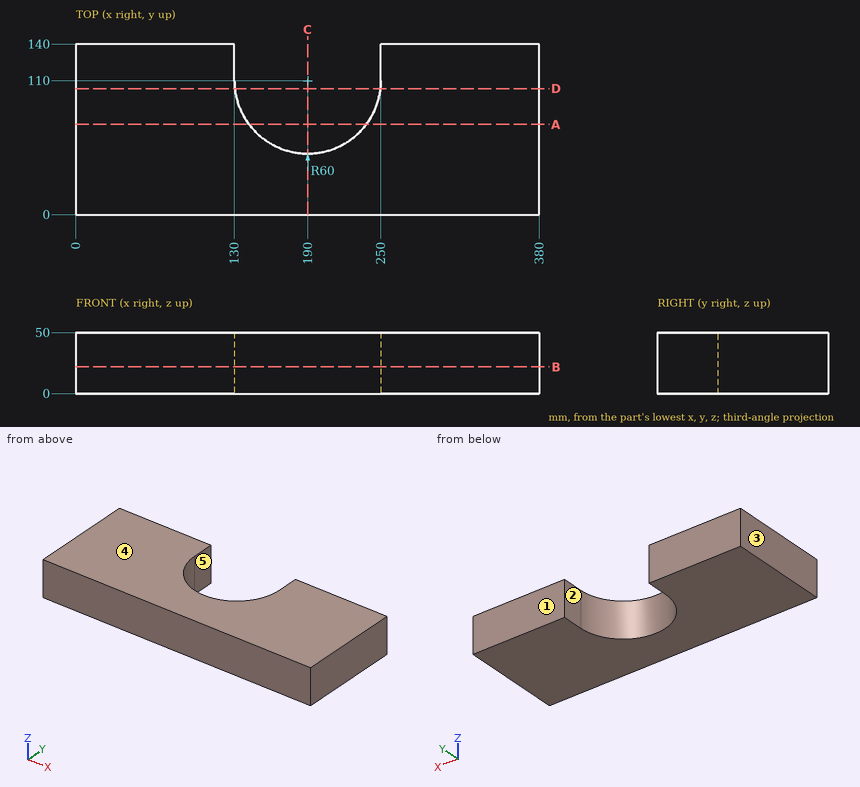
Input: dimensioned drawing with shaded views. Units: mm. Origin: part minimum x, y, z. A direction names the side the tool comes from. Coordinates: 2 decimals unless noted, no trailing zeros. Loops run counter-clockwise (first coordinate to the right, second up) from the corner with the lowest first, then second, coordinate; pieces in that order, holes last. Notation, with made-up numbers: M -32.75,53 L 13.25,53 A16 ccw 13.25,61 Z; hole C 71,48 d10. An arc over 180 degrees is marked long. Use a Markdown table: item, result. Add a question column.
1) Draft query along X for the marked faces 1, 2 and 3. Return one class per face: +X half, -X half, draft (parallel to the pull), parting line (faces both ways), or undercut.
2) Section A-A, the plane y = 74. Return the cut outline in (x, z), plus the area to 3 significant figures.
3) Section B-B, the plane z = 22. Return the cut outline in (x, y), plus the area to 3 significant figures.
4) Section D-D, the plane y = 103.5. Return the cut outline in (x, z), plus the area to 3 significant figures.
5) Set-up query: the marked faces 4 and 5. Return all of +Z, -Z, +X, -X, +Y, -Y with unobstructed straight access to the full face (end or side cutting, diameter ignored); none if empty.
6) Line query: L1, parallel to X at y = 130, z = 42; L2, parallel to X at y = 55, z = 42; L3, parallel to Y at x = 194.5, z = 3. Output: solid intervals per line, ascending. Write a range as from..to.
7) Section C-C, the plane x = 190. Return the cut outline in (y, z), plus the area to 3 significant figures.
Answer below:
| question | item | result |
|---|---|---|
| 1 | face 1 | draft |
| 1 | face 2 | undercut |
| 1 | face 3 | -X half |
| 2 | outline | M 0,0 L 142,0 L 142,50 L 0,50 Z; M 238,0 L 380,0 L 380,50 L 238,50 Z |
| 2 | area | 14,200 mm2 |
| 3 | outline | M 0,0 L 380,0 L 380,140 L 250,140 L 250,110 A60 cw 130,110 L 130,140 L 0,140 Z |
| 3 | area | 43,900 mm2 |
| 4 | outline | M 0,0 L 130.35,0 L 130.35,50 L 0,50 Z; M 249.65,0 L 380,0 L 380,50 L 249.65,50 Z |
| 4 | area | 13,000 mm2 |
| 5 | face 4 | +Z, +X, -X, +Y, -Y |
| 5 | face 5 | +Z, -Z, +Y |
| 6 | L1 | 0..130, 250..380 |
| 6 | L2 | 0..166.02, 213.98..380 |
| 6 | L3 | 0..50.17 |
| 7 | outline | M 0,0 L 50,0 L 50,50 L 0,50 Z |
| 7 | area | 2,500 mm2 |
